from build123d import *

# Parameters (mm, degrees)
CYLINDER_R        = 5
CYLINDER_DEPTH    = 10
CYLINDER004_R     = 5
CYLINDER004_DEPTH = 10
CYLINDER005_R     = 5
CYLINDER005_DEPTH = 10
BOX002_W          = 220
BOX002_H          = 20
BOX002_DEPTH      = 10


with BuildPart() as cilindro:
    # Cylinder → Cylinder (new body)
    with BuildSketch(Plane.XY):
        Circle(CYLINDER_R)
    extrude(amount=CYLINDER_DEPTH)


with BuildPart() as cilindro004:
    # Cylinder004 → Cylinder004 (new body)
    with BuildSketch(Plane(origin=(-98, 0, 4), x_dir=(1, 0, 0), z_dir=(0, 0, 1))):
        Circle(CYLINDER004_R)
    extrude(amount=CYLINDER004_DEPTH)


with BuildPart() as cilindro005:
    # Cylinder005 → Cylinder005 (new body)
    with BuildSketch(Plane(origin=(98, 0, 4), x_dir=(1, 0, 0), z_dir=(0, 0, 1))):
        Circle(CYLINDER005_R)
    extrude(amount=CYLINDER005_DEPTH)


with BuildPart() as obj1:
    # Box002 → Box002 (new body)
    with BuildSketch(Plane(origin=(-110, -10, 0), x_dir=(1, 0, 0), z_dir=(0, 0, 1))):
        with Locations((110, 10)):
            Rectangle(BOX002_W, BOX002_H)
    extrude(amount=BOX002_DEPTH)

    # Cut004: cut Cilindro005
    add(cilindro005.part, mode=Mode.SUBTRACT)

    # Cut005: cut Cilindro004
    add(cilindro004.part, mode=Mode.SUBTRACT)

    # Cut: cut Cilindro
    add(cilindro.part, mode=Mode.SUBTRACT)


solid = obj1.part
Geometry: final body of the model. Coordinates: model frame, mm. A direction names the side the tool comes from. Round coordinates to 2 decimals unless told otherwise and drop trailing zeros. Order: outer loops, then holes, each group sorted by start corner. A loop starts at its lowest first (then second) coordinate and runs counter-clockwise, first axis right, second up.
Q1. Section A-A, the plane x = 0. Output: boundary loops of the cut face in (y, z), and give its area (3 significant figures).
Result sheet:
outline: (-10, 0) - (-5, 0) - (-5, 10) - (-10, 10) - close; (5, 0) - (10, 0) - (10, 10) - (5, 10) - close
area: 100 mm2
Q2. Section C-C, the plane z = 7. Output: boundary loops of the cut face in (x, y), and give its area (3 significant figures).
Result sheet:
outline: (-110, -10) - (110, -10) - (110, 10) - (-110, 10) - close; hole circle Ø10 at (-98, 0); hole circle Ø10 at (0, 0); hole circle Ø10 at (98, 0)
area: 4,160 mm2
Q3. Section B-B, the plane y = 0. Output: boundary loops of the cut face in (x, z).
Result sheet:
outline: (-110, 0) - (-5, 0) - (-5, 10) - (-93, 10) - (-93, 4) - (-103, 4) - (-103, 10) - (-110, 10) - close; (5, 0) - (110, 0) - (110, 10) - (103, 10) - (103, 4) - (93, 4) - (93, 10) - (5, 10) - close
Q4. Section D-D, the plane x = 98. Output: boundary loops of the cut face in (y, z), and give its area (3 significant figures).
Result sheet:
outline: (-10, 0) - (10, 0) - (10, 10) - (5, 10) - (5, 4) - (-5, 4) - (-5, 10) - (-10, 10) - close
area: 140 mm2
Q5. Access query for faces 4 (the face through (98, 0, 4)), 5 (the face through (-2, 7, 0)). Directions: +Z, -Z, +X, -X, +Y, -Y. A direction counts if a zero-diameter tool reaches every point of the face in a straight line with its end or side. Return the directions, or none.
Result sheet:
face 4: +Z
face 5: -Z, +X, -X, +Y, -Y
Q6. Mould query, pull axis Y, two halves, no side actions, for faces 1 (the face through (-110, 0, 5)), 2 (the face through (-2, 10, 5)), 3 (the face through (-98, 0, 4)). Classes: released by +Y, released by -Y, zero draft, split by the parting line, or undercut.
Result sheet:
face 1: zero draft
face 2: released by +Y
face 3: undercut
Q7. Pin query (flat end, axial travel): pin 1 (5 mm diameter, centred on x = 96, y = -0.5, fed in from +Z). Return the tip coordinate at first contact, or that it passes through.
Result sheet:
pin 1: stops at z = 4
Q8. Material intervals for probe 1 along Y at (x, z) = (-98, 5.65); probe 2 along X at (y, z) = (1.5, 8.25); probe 3 along X at (y, z) = (-0.25, 2), sorted ascending.
Result sheet:
probe 1: y = -10 to -5, 5 to 10
probe 2: x = -110 to -102.77, -93.23 to -4.77, 4.77 to 93.23, 102.77 to 110
probe 3: x = -110 to -4.99, 4.99 to 110
